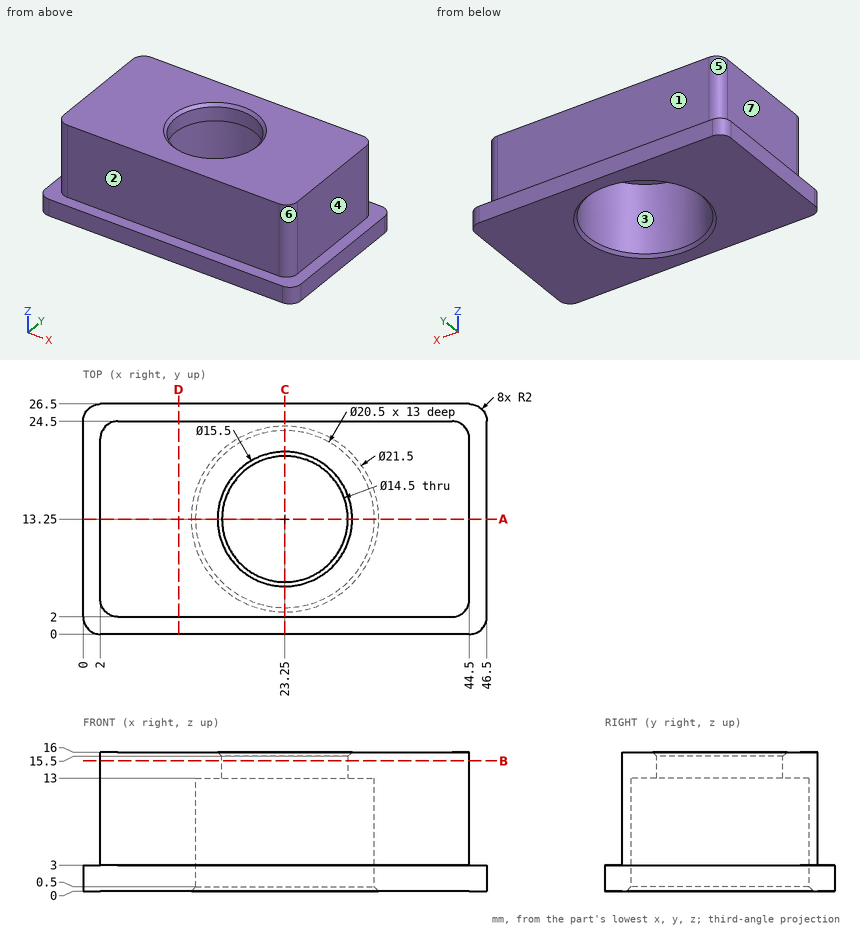
Answer from the drawing. Dimensions are ordinates in mm from the lowest x, y and z of the part. A direction names the side the tool comes from. Give positions to 0.01 mm unless a question says otherwise; leave off trailing zeros. Loops run counter-clockwise (first coordinate to the right, second up) from the corner with the lowest first, then second, coordinate; pieces in that order, holes last.
Item 1: The part is cut by section A-A (y = 13.25). Write down the section's boundary in (x, z).
Item 2: The mould has two halves that part along Y. Classify the marked faces 1, 2 and 3: released by +Y, released by -Y, zero draft, split by the parting line, or undercut.
Item 3: Find the intervals of material crossed by line 1 along Y through (x, z) = (23.25, 14.5); line 2 along Y through (x, z) = (23.25, 10.25); line 3 along Z through (x, y) = (24, 25.5), in increasing order.
Item 4: Each of these flat-tipped pins is pushed along its axis until it touches: pin 1 Ø8 at (x, z) = (16.5, 14) entering from +Y; pin 2 Ø10 at (x, y) = (23.5, 9.5) entering from +Z; pin 3 Ø6.5 at (y, z) = (16, 9.5) entering from +X; pin 4 Ø2 at (x, z) = (40.5, 13.5) entering from -Y. Where does it stop, or does it pass through?
Item 5: The part is cut by section D-D (x = 11). Write down the section's boundary in (y, z).
Item 6: For the marked faces 4, 5, 6 and 7, determine the directions among +Z, -Z, +X, -X, +Y, -Y from which every point of the face is accessible in a straight line to the end or side of a thin tool.
Item 7: The part is cut by section C-C (x = 23.25). Write down the section's boundary in (y, z), and give its area (3 significant figures).
Item 8: The part is cut by section B-B (z = 15). Write down the section's boundary in (x, y).
Taken from the geometry:
1. outline: (0, 0) - (12.5, 0) - (13, 0.5) - (13, 13) - (16, 13) - (16, 15.5) - (15.5, 16) - (2, 16) - (2, 3) - (0, 3) - close; (30.5, 13) - (33.5, 13) - (33.5, 0.5) - (34, 0) - (46.5, 0) - (46.5, 3) - (44.5, 3) - (44.5, 16) - (31, 16) - (30.5, 15.5) - close
2. face 1: released by +Y
2. face 2: released by -Y
2. face 3: undercut
3. line 1: y = 2 to 6, 20.5 to 24.5
3. line 2: y = 2 to 3, 23.5 to 24.5
3. line 3: z = 0 to 3
4. pin 1: stops at y = 24.5
4. pin 2: stops at z = 16
4. pin 3: stops at x = 44.5
4. pin 4: stops at y = 2
5. outline: (0, 0) - (26.5, 0) - (26.5, 3) - (24.5, 3) - (24.5, 16) - (2, 16) - (2, 3) - (0, 3) - close
6. face 4: +Z, +X, +Y, -Y
6. face 5: +Z, -X, +Y
6. face 6: +Z, +X, -Y
6. face 7: +Z, -X, +Y, -Y
7. outline: (0, 0) - (2.5, 0) - (3, 0.5) - (3, 13) - (6, 13) - (6, 15.5) - (5.5, 16) - (2, 16) - (2, 3) - (0, 3) - close; (20.5, 13) - (23.5, 13) - (23.5, 0.5) - (24, 0) - (26.5, 0) - (26.5, 3) - (24.5, 3) - (24.5, 16) - (21, 16) - (20.5, 15.5) - close
7. area: 61.5 mm2
8. outline: (2, 4) arc R2 ccw to (4, 2) - (42.5, 2) arc R2 ccw to (44.5, 4) - (44.5, 22.5) arc R2 ccw to (42.5, 24.5) - (4, 24.5) arc R2 ccw to (2, 22.5) - close; hole circle Ø14.5 at (23.25, 13.25)
